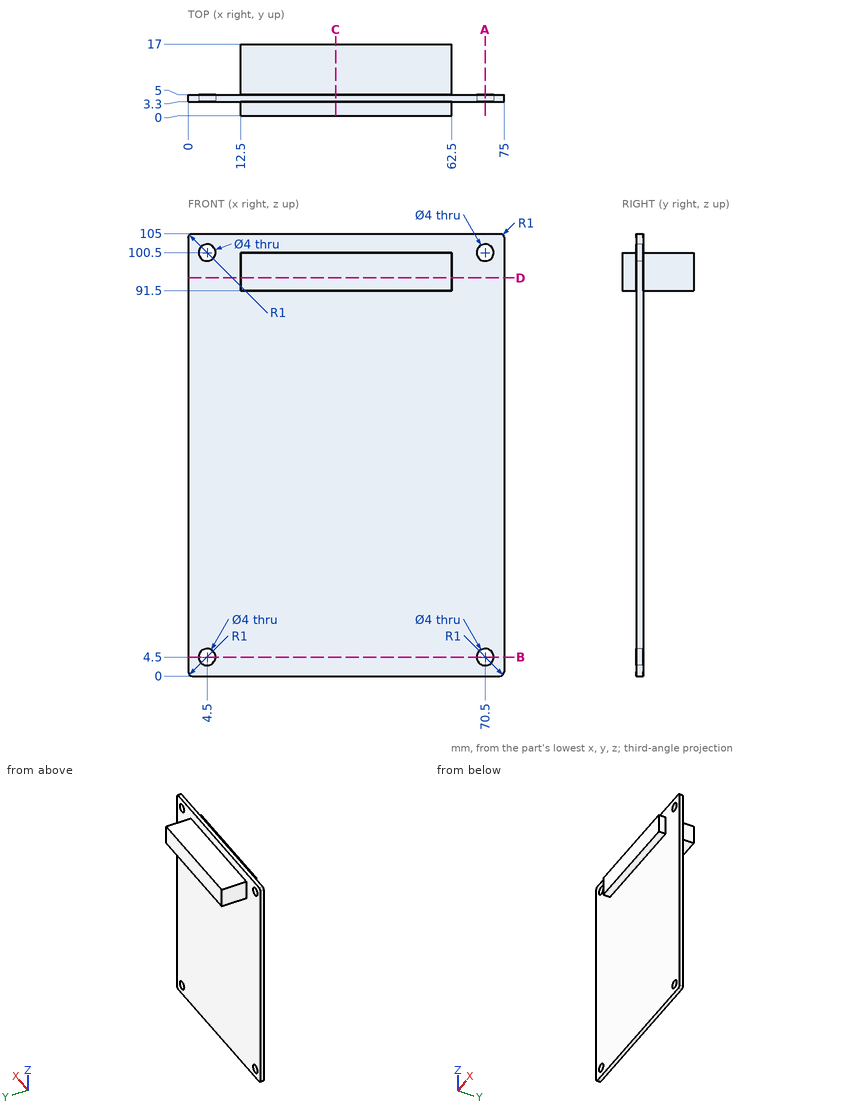
Study the drawing (mm; zero at the part's minimum x, y, z) and answer. Coordinates: 2 decimals unless noted, no trailing zeros. Write each loop counter-clockwise with the first axis right and the second up, starting at its lowest first coordinate (ties: lowest second). Pieces come first, ordered by that corner, then holes. Notation, with made-up numbers: (10, -7.75) - (51, -7.75) arc R23 ccw to (51, 13.25) - close; hole circle Ø3 at (12, -38.75). An arc over 180 degrees is marked (long way). Return JSON: item names as keys, results as strings. Group by question number.
1. Straight lines are drawn through the part: L1, parallel to Z at x = 70.5, y = 3.7; L2, parallel to Y at x = 28, z = 45; L3, parallel to Z at x = 46, y = 9.25. For each, find the intervals that lie inside material, in ascending order.
2. A cutting plane is placed at D-D, the plane z = 94.5. Determine the outline of the cut face in (x, y).
3. A cutting plane is placed at A-A, the plane x = 70.5. Determine the outline of the cut face in (y, z), plus the area to 3 significant figures.
4. A cutting plane is placed at B-B, the plane z = 4.5. Determine the outline of the cut face in (x, y), plus the area to 3 significant figures.
5. A cutting plane is placed at C-C, the plane x = 35. Determine the outline of the cut face in (y, z), plus the area to 3 significant figures.
6. Given pin 1 (2.5 mm diameter, centred on x = 70.5, z = 4.5, fed in from -Y); pin 2 (1 mm diameter, centred on x = 38, y = 1, fed in from +Z); pin 3 (2.5 mm diameter, centred on y = 1.5, z = 96.5, fed in from +X); pin 4 (1.6 mm diameter, centred on x = 42.5, y = 2, fed in from -Z), each flat-ended and moving along its own axis, determine where each tip first touches the part or whether it passes through.
Ans:
{
 "1": {"L1": "0 to 2.5, 6.5 to 98.5, 102.5 to 105", "L2": "3.3 to 5", "L3": "91.5 to 100.5"},
 "2": {"outline": "(0, 3.3) - (12.5, 3.3) - (12.5, 0) - (62.5, 0) - (62.5, 3.3) - (75, 3.3) - (75, 5) - (62.5, 5) - (62.5, 17) - (12.5, 17) - (12.5, 5) - (0, 5) - close"},
 "3": {"outline": "(3.3, 0) - (5, 0) - (5, 2.5) - (3.3, 2.5) - close; (3.3, 6.5) - (5, 6.5) - (5, 98.5) - (3.3, 98.5) - close; (3.3, 102.5) - (5, 102.5) - (5, 105) - (3.3, 105) - close", "area": "165 mm²"},
 "4": {"outline": "(0, 3.3) - (2.5, 3.3) - (2.5, 5) - (0, 5) - close; (6.5, 3.3) - (68.5, 3.3) - (68.5, 5) - (6.5, 5) - close; (72.5, 3.3) - (75, 3.3) - (75, 5) - (72.5, 5) - close", "area": "114 mm²"},
 "5": {"outline": "(0, 91.5) - (3.3, 91.5) - (3.3, 0) - (5, 0) - (5, 91.5) - (17, 91.5) - (17, 100.5) - (5, 100.5) - (5, 105) - (3.3, 105) - (3.3, 100.5) - (0, 100.5) - close", "area": "316 mm²"},
 "6": {"pin 1": "through", "pin 2": "z = 100.5", "pin 3": "x = 62.5", "pin 4": "z = 91.5"}
}
